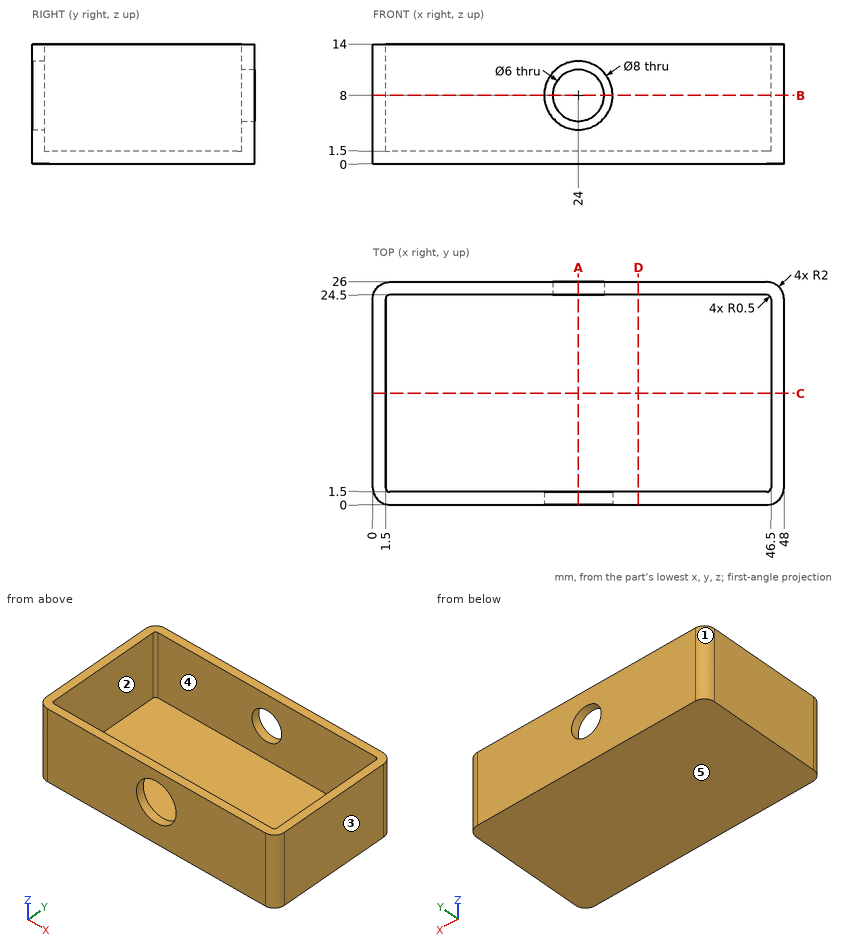
Study the drawing (mm; zero at the part's minimum x, y, z) and answer. A direction names the side the tool comes from. Round coordinates to 2 decimals unless told otherwise and drop trailing zeros. Write each loop counter-clockwise with the first axis right and the second up, starting at its lowest first coordinate (ties: lowest second). Pieces come first, ordered by that corner, then holes. Notation, with made-up numbers: (51.5, 63) -> (78.5, 63) arc R15 ccw to (78.5, 78) -> close; hole circle Ø2 at (69.5, 30). An arc over 180 degrees is marked (long way). Answer as CSV lines item,"result". Start each with the question number.
(1) The part is cut by section D-D, the plane x = 31. Give the vertices of the cut face in (y, z).
(2) Each of these flat-tipped pins is pushed along its axis until it touches: pin 1 (6 mm diameter, centred on x = 42.5, y = 7.5, fed in from +Z); pin 2 (5 mm diameter, centred on x = 24, z = 8, fed in from -Y). Where does it stop, or does it pass through?
(3) The part is cut by section B-B, the plane z = 8. Give the vertices of the cut face in (x, y).
(4) The part is cut by section C-C, the plane y = 13. Give the vertices of the cut face in (x, z), then the cut area to 4 significant figures.
(5) The mould has two halves that part along X. Classify the marked faces 3, 4 and 5: +X half, -X half, draft (parallel to the pull), parting line (faces both ways), or undercut.
(6) The part is cut by section A-A, the plane x = 24. Give the vertices of the cut face in (y, z).
(7) Find the intervals of material crossed by probe 1 along Y at (x, z) = (21.5, 11.75); probe 2 along X at (y, z) = (3, 5); probe 3 along X at (y, z) = (25.25, 8), in increasing order.
(8) A tool of negligible diameter and unlimited length cuts with its end or side. For the marked faces 1 and 2, from which of +Z, -Z, +X, -X, +Y, -Y can it reach the whole face along a straight path? Write none if from no direction.
Output values:
1,outline,"(0, 0) -> (26, 0) -> (26, 14) -> (24.5, 14) -> (24.5, 1.5) -> (1.5, 1.5) -> (1.5, 14) -> (0, 14) -> close"
2,pin 1,"stops at z = 1.5"
2,pin 2,"passes through"
3,outline,"(0, 2) arc R2 ccw to (2, 0) -> (20, 0) -> (20, 1.5) -> (2, 1.5) arc R0.5 cw to (1.5, 2) -> (1.5, 24) arc R0.5 cw to (2, 24.5) -> (21, 24.5) -> (21, 26) -> (2, 26) arc R2 ccw to (0, 24) -> close; (27, 24.5) -> (46, 24.5) arc R0.5 cw to (46.5, 24) -> (46.5, 2) arc R0.5 cw to (46, 1.5) -> (28, 1.5) -> (28, 0) -> (46, 0) arc R2 ccw to (48, 2) -> (48, 24) arc R2 ccw to (46, 26) -> (27, 26) -> close"
4,outline,"(0, 0) -> (48, 0) -> (48, 14) -> (46.5, 14) -> (46.5, 1.5) -> (1.5, 1.5) -> (1.5, 14) -> (0, 14) -> close"
4,area,"109.5 mm²"
5,face 3,"+X half"
5,face 4,"undercut"
5,face 5,"draft"
6,outline,"(0, 0) -> (26, 0) -> (26, 5) -> (24.5, 5) -> (24.5, 1.5) -> (1.5, 1.5) -> (1.5, 4) -> (0, 4) -> close; (0, 12) -> (1.5, 12) -> (1.5, 14) -> (0, 14) -> close; (24.5, 11) -> (26, 11) -> (26, 14) -> (24.5, 14) -> close"
7,probe 1,"y = 0 to 1.5, 24.5 to 26"
7,probe 2,"x = 0 to 1.5, 46.5 to 48"
7,probe 3,"x = 0.44 to 21, 27 to 47.56"
8,face 1,"+Z, -Z, -X, +Y"
8,face 2,"+Z"
